```python
from build123d import *

# Parameters (mm, degrees)
SKETCH_1_W           = 10
SKETCH_1_H           = 6
EXTRUDE_1_DEPTH      = 7.5
SHELL_1_T            = -0.5
SKETCH_2_W           = 13.621733733
SKETCH_2_H           = 0.5
SKETCH_2_W_2         = 1
SKETCH_2_H_2         = 1.110036837
CUT_EXTRUDE_1_DEPTH  = 3.5
EXTRUDE_2_DEPTH      = 6.5
EXTRUDE_2_DEPTH_BACK = 3
SKETCH_3_W           = 0.5
SKETCH_3_H           = 0.5


with BuildPart() as part:
    # 草图1 → 凸台-拉伸1 (new body)
    with BuildSketch(Plane(origin=(0, 0, 0), x_dir=(1, 0, 0), z_dir=(0, 1, 0))):
        Rectangle(SKETCH_1_W, SKETCH_1_H)
    extrude(amount=EXTRUDE_1_DEPTH)

    # 抽壳1
    shell_1_openings = [part.faces().sort_by_distance(p)[0] for p in [
        (0, 7.5, 0),
    ]]
    offset(amount=SHELL_1_T, openings=shell_1_openings, kind=Kind.INTERSECTION)

    # 草图2 → 切除-拉伸1 (cut)
    with BuildSketch(Plane(origin=(0, 7.5, 0), x_dir=(1, 0, 0), z_dir=(0, 1, 0))):
        with Locations((0.222754883, -2.249)):
            Rectangle(SKETCH_2_W, SKETCH_2_H)
        with Locations((-2.5, -3.055018419)):
            Rectangle(SKETCH_2_W_2, SKETCH_2_H_2)
        with Locations((2.5, -3.055018419)):
            Rectangle(SKETCH_2_W_2, SKETCH_2_H_2)
    extrude(amount=-CUT_EXTRUDE_1_DEPTH, mode=Mode.SUBTRACT)

    # 草图3 → 凸台-拉伸2 (add, two sides: drawn at the far end of the back side and taken through both)
    with BuildSketch(Plane(origin=(0, 0.5, 0), x_dir=(1, 0, 0), z_dir=(0, 1, 0)).offset(-EXTRUDE_2_DEPTH_BACK)):
        with Locations((0, -0.5)):
            Rectangle(SKETCH_3_W, SKETCH_3_H)
        with Locations((-2.5, -0.5)):
            Rectangle(SKETCH_3_W, SKETCH_3_H)
        with Locations((2.5, -0.5)):
            Rectangle(SKETCH_3_W, SKETCH_3_H)
    extrude(amount=EXTRUDE_2_DEPTH + EXTRUDE_2_DEPTH_BACK)


solid = part.part
```
Here's how the part is built. I have some questions about the finished solid (model axes, mm). A direction names the side the tool comes from. Give positions to 0.01 mm unless a question says otherwise; leave off trailing zeros. Write each loop counter-clockwise with the first axis right and the second up, starting at its lowest first coordinate (ties: lowest second). Pieces come first, ordered by that corner, then holes. Notation, with made-up numbers: (26, 54) -> (61, 54) arc R10 cw to (61, 68) -> close; hole circle Ø6 at (15, 77). An arc over 180 degrees is marked (long way). Write each question's results on one line, items separated by ' | '.
Item 1: Suppose I cut it at A-A on y = 3.5. Write out the boundary of the cut face in (x, z).
Output:
outline: (-5, -3) -> (5, -3) -> (5, 3) -> (-5, 3) -> close; (-2.75, 0.25) -> (-2.25, 0.25) -> (-2.25, 0.75) -> (-2.75, 0.75) -> close; (-0.25, 0.25) -> (0.25, 0.25) -> (0.25, 0.75) -> (-0.25, 0.75) -> close; (2.25, 0.25) -> (2.75, 0.25) -> (2.75, 0.75) -> (2.25, 0.75) -> close; hole (-4.5, -2.5) -> (4.5, -2.5) -> (4.5, 2.5) -> (-4.5, 2.5) -> close
Item 2: Suppose I cut it at D-D on z = -0.4. Write out the boundary of the cut face in (x, y), plus the area to 3 significant figures.
Output:
outline: (-5, 0) -> (5, 0) -> (5, 7.5) -> (4.5, 7.5) -> (4.5, 0.5) -> (-4.5, 0.5) -> (-4.5, 7.5) -> (-5, 7.5) -> close | area: 12.0 mm^2
Item 3: Suppose I cut it at C-C on y = -1. Write out the boundary of the cut face in (x, z).
Output:
outline: (-2.75, 0.25) -> (-2.25, 0.25) -> (-2.25, 0.75) -> (-2.75, 0.75) -> close; (-0.25, 0.25) -> (0.25, 0.25) -> (0.25, 0.75) -> (-0.25, 0.75) -> close; (2.25, 0.25) -> (2.75, 0.25) -> (2.75, 0.75) -> (2.25, 0.75) -> close
Item 4: We'd pull the mould along Z, two halves only. Please class faces 3 (the face through (0, 4, -3)), 4 (the face through (0, 0, 0)), 5 (the face through (0, 4, 2.5)): pulls with the +Z half, pulls with the -Z half, needs draft (parallel to the pull), parting line crosses it, or undercut.
Output:
face 3: pulls with the -Z half | face 4: needs draft | face 5: undercut
Item 5: Suppose I cut it at B-B on x = 0. Write out the boundary of the cut face in (y, z), plus the area to 3 significant figures.
Output:
outline: (-2.5, 0.25) -> (0, 0.25) -> (0, -3) -> (7.5, -3) -> (7.5, -2.5) -> (0.5, -2.5) -> (0.5, 0.25) -> (7, 0.25) -> (7, 0.75) -> (0.5, 0.75) -> (0.5, 2.5) -> (7.5, 2.5) -> (7.5, 3) -> (0, 3) -> (0, 0.75) -> (-2.5, 0.75) -> close | area: 14.5 mm^2
Item 6: For pin 1 Ø2 at (x, z) = (-2.5, 1) entering from -Y; pin 2 Ø0.5 at (x, z) = (2.5, 3) entering from +Y; pin 3 Ø0.6 at (y, z) = (-2, 0.5) entering from +X, each with a flat end and sliding along its axis, tell me the tip position at first contact or that it passes through.
Output:
pin 1: stops at y = -2.5 | pin 2: stops at y = 4 | pin 3: stops at x = 2.75
Item 7: On a 3-axis mill with a long thin cutter (end or side, diameter ignored), from which of +Z, -Z, +X, -X, +Y, -Y can I reach the whole of each face in a straight line? I mean faces 1 (the face through (4.5, 4, 0)), 2 (the face through (-5, 4, 0)). Say none if no direction works.
Output:
face 1: +Y | face 2: +Z, -Z, -X, +Y, -Y
Item 8: If I drill on L1, parallel to X at y = -0.5, z = 0.3; L2, parallel to X at y = 0.75, z = 0.45; L3, parallel to X at y = 4.5, z = 2.65, over which ranges is the centre line in solid material (lowest first)?
Output:
L1: x = -2.75 to -2.25, -0.25 to 0.25, 2.25 to 2.75 | L2: x = -5 to -4.5, -2.75 to -2.25, -0.25 to 0.25, 2.25 to 2.75, 4.5 to 5 | L3: x = -5 to -3, -2 to 2, 3 to 5
